For this review, use the dimensioned drawing (mm, ordinates from the lowest corner) and the shaded views. A direction names the side the tool comes from. Coordinates: 2 decimals unless noted, no trailing zeros. Loops run counter-clockwise (first coordinate to the right, second up) from the corner with the lowest first, then second, coordinate; pieces in that order, holes last. Notation, with made-up numbers: M 69,-9.75 L 90,-9.75 A33 cw 90,23.25 Z; hole C -10.5,89.25 d9. An arc over 180 degrees is marked long. One line per item, written item: value.
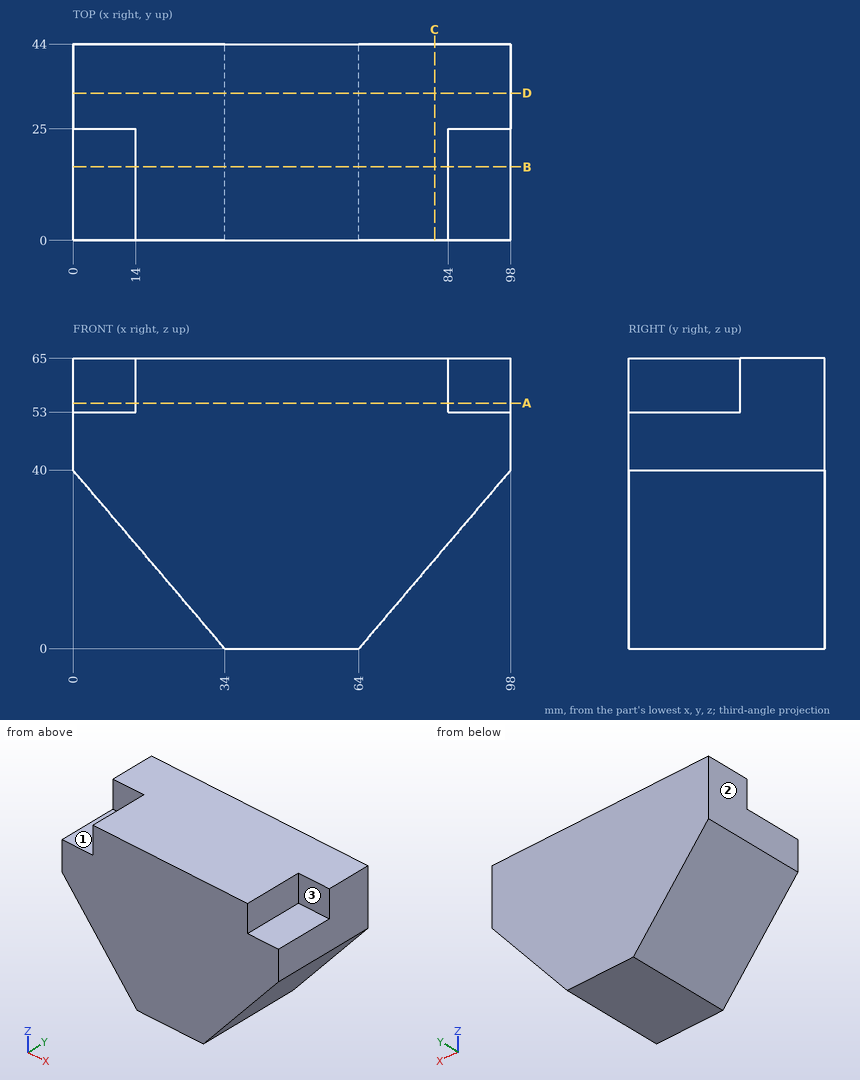
(1) Tool access review of the marked faces 1, 2 and 3: name each direction out of +Z, -Z, +X, -X, +Y, -Y from which nothing blocks a thin tool from reaching the whole face with its end or side.
Checks:
face 1: +Z, -X, -Y
face 2: +Z, -Z, -X, +Y, -Y
face 3: +Z, +X, -Y
(2) Add section D-D on y = 33. State the section outline as (x, z) points, then the cut area to 3 significant figures.
Checks:
outline: M 0,40 L 34,0 L 64,0 L 98,40 L 98,65 L 0,65 Z
area: 5,010 mm^2
(3) To check wall thickness, follow L1, parallel to X at y = 2, z = 62.5; L2, parallel to X at y = 12, z = 3.5 (3 decimals); L3, parallel to Z at x = 27, y = 12.5. State the ranges of each line that lie inside material, in increasing order. Write a range as [from, to].
Checks:
L1: [14, 84]
L2: [31.025, 66.975]
L3: [8.24, 65]
(4) Add section B-B on y = 16.5. State the section outline as (x, z) points.
Checks:
outline: M 0,40 L 34,0 L 64,0 L 98,40 L 98,53 L 84,53 L 84,65 L 14,65 L 14,53 L 0,53 Z
(5) Add section C-C on x = 81. State the section outline as (y, z) points.
Checks:
outline: M 0,20 L 44,20 L 44,65 L 0,65 Z
(6) Insertion check: pin 1 Ø6 at (y, z) = (17, 25) entering from -X; pin 2 Ø6 at (x, z) = (91.5, 61.5) entering from -Y; pin 3 Ø11 at (x, y) = (4, 12) entering from +Z. Each pin has a flat end and moves straight along its axis. Give the tip position at first contact, or say it passes through.
Checks:
pin 1: x = 10.2
pin 2: y = 25
pin 3: z = 53
(7) Add section A-A on z = 55. State the section outline as (x, y) points.
Checks:
outline: M 0,25 L 14,25 L 14,0 L 84,0 L 84,25 L 98,25 L 98,44 L 0,44 Z
